```python
from build123d import *

# Parameters (mm, degrees)
SKETCH1_R           = 80
SKETCH1_R_2         = 1.5
SKETCH1_W           = 17
SKETCH1_H           = 65
SKETCH1_W_2         = 5
SKETCH1_H_2         = 21
SKETCH1_H_3         = 12
SKETCH1_W_3         = 20
SKETCH1_H_4         = 5
BOSS_EXTRUDE1_DEPTH = 5
SKETCH2_R           = 1.5
SKETCH2_W           = 16
SKETCH2_H           = 8.5
SAFETY_LINK_DEPTH   = 10


with BuildPart() as part:
    # Sketch1 → Boss-Extrude1 (new body)
    with BuildSketch(Plane(origin=(0, 0, 0), x_dir=(1, 0, 0), z_dir=(0, 1, 0))):
        with Locations(Location((0, 0, 0), (0, 0, 270))):
            Circle(SKETCH1_R)
        with Locations(Location((-6, 71, 0), (0, 0, 270))):
            Circle(SKETCH1_R_2, mode=Mode.SUBTRACT)
        with Locations(Location((6, 49, 0), (0, 0, 270))):
            Circle(SKETCH1_R_2, mode=Mode.SUBTRACT)
        with Locations((-57.5, 0)):
            Rectangle(SKETCH1_W, SKETCH1_H, mode=Mode.SUBTRACT)
        with Locations((57.5, 0)):
            Rectangle(SKETCH1_W, SKETCH1_H, mode=Mode.SUBTRACT)
        with Locations((0, 64.5)):
            Rectangle(SKETCH1_W_2, SKETCH1_H_2, mode=Mode.SUBTRACT)
        Polygon((-5.5, 52.5), (0.5, 52.5), (3.144904711, 37.5), (-8.144904711, 37.5), align=None, mode=Mode.SUBTRACT)
        with Locations((42.5, -50.282032303)):
            Rectangle(SKETCH1_W_2, SKETCH1_H_3, mode=Mode.SUBTRACT)
        with Locations((-42.5, -50.282032303)):
            Rectangle(SKETCH1_W_2, SKETCH1_H_3, mode=Mode.SUBTRACT)
        with Locations((0, -30.782032303)):
            Rectangle(SKETCH1_W_3, SKETCH1_H_4, mode=Mode.SUBTRACT)
    extrude(amount=BOSS_EXTRUDE1_DEPTH)

    # Sketch2 → safety_link (cut)
    with BuildSketch(Plane(origin=(0, 5, 0), x_dir=(1, 0, 0), z_dir=(0, 1, 0))):
        with Locations(Location((-12, 0, 0), (0, 0, 270))):
            Circle(SKETCH2_R)
        with Locations(Location((12, 0, 0), (0, 0, 270))):
            Circle(SKETCH2_R)
        Rectangle(SKETCH2_W, SKETCH2_H)
    extrude(amount=-SAFETY_LINK_DEPTH, mode=Mode.SUBTRACT)


solid = part.part
```
Check sheet for the modelled part. Datum: model origin and axes. Units: mm. Round coordinates to 2 decimals unless told otherwise and drop trailing zeros. Order: outer loops, then holes, each group sorted by start corner. A loop starts at its lowest first (then second) coordinate and runs counter-clockwise, first axis right, second up. Notation, with made-up numbers: M 32.25,38.25 L 62.25,38.25 A15 ccw 62.25,59.25 Z; hole C 70,-22 d2. An arc over 180 degrees is marked long. Answer in a Markdown table with one row per item.
(1) Section check A-A on x = 54. Record the boundary of the cut face in (y, z).
Findings:
| item | result |
|---|---|
| outline | M 0,-59.03 L 5,-59.03 L 5,-32.5 L 0,-32.5 Z; M 0,32.5 L 5,32.5 L 5,59.03 L 0,59.03 Z |
(2) Material ranges on line 1 along X through (y, z) = (1.55, 0); line 2 along X through (y, z) = (4.7, -10); line 3 along X through (y, z) = (2.6, 1), recorded low to high. Write a range as from..to.
Findings:
| item | result |
|---|---|
| line 1 | x = -80..-66, -49..-13.5, -10.5..-8, 8..10.5, 13.5..49, 66..80 |
| line 2 | x = -79.37..-66, -49..49, 66..79.37 |
| line 3 | x = -79.99..-66, -49..-13.12, -10.88..-8, 8..10.88, 13.12..49, 66..79.99 |
(3) Draft check along Z on faces 1 (the flat face through (1, 5, 17)), 2 (the flat face through (-49, 2, 0)), 3 (the cylindrical face through (-78.1, 2.46, -17.34)). Enter one of: +Z half, -Z half, draft (parallel to the pull), parting line (faces both ways), or undercut.
Findings:
| item | result |
|---|---|
| face 1 | draft |
| face 2 | undercut |
| face 3 | parting line |
(4) Gauge pin test, flat ends, axial feed: pin 1 (1.5 mm diameter, centred on y = 1, z = 39.5, fed in from +X); pin 2 (2.5 mm diameter, centred on y = 2, z = -1, fed in from +X); pin 3 (1.5 mm diameter, centred on x = 41.5, y = 1.5, fed in from +Z); pin 4 (3 mm diameter, centred on x = 1.5, z = 26, fed in from -Y). Record the tip position at first contact, or that the pin passes through.
Findings:
| item | result |
|---|---|
| pin 1 | stops at x = 69.99 |
| pin 2 | stops at x = 80 |
| pin 3 | stops at z = 68.84 |
| pin 4 | stops at y = 0 |
(5) Section check B-B on z = 22.5. Record the boundary of the cut face in (x, y), plus the area to 3 significant figures.
Findings:
| item | result |
|---|---|
| outline | M -76.77,0 L -66,0 L -66,5 L -76.77,5 Z; M -49,0 L 49,0 L 49,5 L -49,5 Z; M 66,0 L 76.77,0 L 76.77,5 L 66,5 Z |
| area | 598 mm^2 |
(6) Section check D-D on y = 1.9. Give the number of separate pieces and of enclosed holes in the cut face, plus the area to 3 significant figures.
Findings:
| item | result |
|---|---|
| separate pieces | 1 |
| enclosed holes | 12 |
| area | 17,300 mm^2 |
(7) Section check C-C on x = -62. Record the boundary of the cut face in (y, z), plus the area to 3 significant figures.
Findings:
| item | result |
|---|---|
| outline | M 0,-50.56 L 5,-50.56 L 5,-32.5 L 0,-32.5 Z; M 0,32.5 L 5,32.5 L 5,50.56 L 0,50.56 Z |
| area | 181 mm^2 |
